Can you work these out from the model? Positions are in its coordinate system, mm. Round coordinates to 2 decimals unless told otherwise and drop trailing zeros. Loops run counter-clockwise (first coordinate to the right, second up) from the corner with the lowest first, then second, coordinate; pieces in that order, holes last.
from build123d import *

# Parameters (mm, degrees)
BOSS_EXTRUDE1_DEPTH     = 1.5875
CUT_EXTRUDE1_DEPTH      = 16.380616986
CUT_EXTRUDE1_DEPTH_BACK = 16.380616986
SKETCH2_R               = 1.75
FILLET1_R               = 1
FILLET2_R               = 5


with BuildPart() as part:
    # Sketch1 → Boss-Extrude1 (new, symmetric)
    with BuildSketch(Plane.XY):
        Polygon((11.81540086, -9.32089354), (3.370357256, 9.32089354), (-11.81540086, 9.32089354), (-11.81540086, -9.32089354), align=None)
    extrude(amount=BOSS_EXTRUDE1_DEPTH, both=True)

    # Sketch2 → Cut-Extrude1 (cut, two sides: drawn at the far end of the back side and taken through both)
    with BuildSketch(Plane.XY.offset(1.5875).offset(-CUT_EXTRUDE1_DEPTH_BACK)):
        with Locations(Location((0.195357254, -0.67910646, 0), (0, 0, 180))):
            Circle(SKETCH2_R)
        with Locations((-8.640400858, -0.67910646)):
            Circle(SKETCH2_R)
    extrude(amount=CUT_EXTRUDE1_DEPTH + CUT_EXTRUDE1_DEPTH_BACK, mode=Mode.SUBTRACT)

    # Fillet1
    fillet1_edges = [part.edges().sort_by_distance(p)[0] for p in [
        (3.370357256, 9.32089354, 0),
        (11.81540086, -9.32089354, 0),
    ]]
    fillet(fillet1_edges, radius=FILLET1_R)

    # Fillet2
    fillet2_edges = [part.edges().sort_by_distance(p)[0] for p in [
        (-11.81540086, -9.32089354, 0),
        (-11.81540086, 9.32089354, 0),
    ]]
    fillet(fillet2_edges, radius=FILLET2_R)


solid = part.part
(1) If we section it at C-C, the plane x = 0.75: List the corners of the cut face in (y, z) for me.
Worked answers:
outline: (-9.32, -1.59) - (-2.34, -1.59) - (-2.34, 1.59) - (-9.32, 1.59) - close; (0.98, -1.59) - (9.32, -1.59) - (9.32, 1.59) - (0.98, 1.59) - close
(2) If we section it at A-A, the plane x = -9.5: List the corners of the cut face in (y, z) for me.
Worked answers:
outline: (-8.54, -1.59) - (-2.2, -1.59) - (-2.2, 1.59) - (-8.54, 1.59) - close; (0.85, -1.59) - (8.54, -1.59) - (8.54, 1.59) - (0.85, 1.59) - close
(3) Will these pins go through, and if not, where does the flat tip stop? P1, Ø4, axis at x = 0.2, y = -0.68, coming from the -Z side; P2, Ø2, axis at x = -8.64, y = -0.68, coming from the +Z side.
Worked answers:
P1: stops at z = -1.59
P2: passes through
(4) If we section it at D-D, the plane y = -5.5: List the corners of the cut face in (x, z) for me, then the cut area to 3 significant figures.
Worked answers:
outline: (-11.67, -1.59) - (10.08, -1.59) - (10.08, 1.59) - (-11.67, 1.59) - close
area: 69.1 mm2
(5) If we section it at B-B, the plane z = 0: List the corners of the cut face in (x, y) for me, then the cut area to 3 significant figures.
Worked answers:
outline: (-11.82, -4.32) arc R5 ccw to (-6.82, -9.32) - (10.26, -9.32) arc R1 ccw to (11.18, -7.91) - (3.64, 8.73) arc R1 ccw to (2.73, 9.32) - (-6.82, 9.32) arc R5 ccw to (-11.82, 4.32) - close; hole circle Ø3.5 at (-8.64, -0.68); hole circle Ø3.5 at (0.2, -0.68)
area: 331 mm2
(6) If I drill on line 1 (Y direction, x = 1.75, z = 0.9); line 2 (Y direction, x = -9, z = -1.1); line 3 (Y direction, x = 9.25, z = 0.2), over which ranges is the centre line in solid material (lowest first)?
Worked answers:
line 1: y = -9.32 to -1.48, 0.12 to 9.32
line 2: y = -8.82 to -2.39, 1.03 to 8.82
line 3: y = -9.32 to -3.66
(7) If we mould it in two halves opening along Y, with no side actions, what happens to faces 1 (the cylindrical face through (-7.83, -2.23, -0.02)), 2 (the cylindrical face through (0.423, -2.414, -0.022)), 3 (the flat face through (-11.815, 0, 0)), 4 (the cylindrical face through (-10.312, -7.895, -0.022))? For each: released by +Y, released by -Y, zero draft, split by the parting line, or undercut.
Worked answers:
face 1: undercut
face 2: undercut
face 3: zero draft
face 4: released by -Y
